The model under review builds one solid part; all positions refer to its coordinate system, in mm. A direction names the side the tool comes from. Coordinates: 2 decimals unless noted, no trailing zeros. Write each loop counter-clockwise with the first axis right and the second up, starting at its lowest first coordinate (ties: lowest second). Pieces come first, ordered by that corner, then holes. Notation, with made-up numbers: (26, 9) - (61, 9) arc R8 cw to (61, 20) - close; hole circle Ø2 at (51, -0.5). An arc over 180 degrees is marked (long way). Return JSON: item names as keys, results as strings. Group by question number.
(1) For pin 1 Ø3 at (x, y) = (108, -9.5) entering from +Z; pin 2 Ø9 at (y, z) = (0.5, -7) entering from +X; pin 3 Ø1 at (x, y) = (56.5, 34) entering from -Z; pin 4 Ø5 at (x, z) = (20, -49.5) entering from +Y, all flat-tipped, find the tip position at first contact; note any pin that passes through.
(2) We need section A-A on y = 0. Give the number of separate pieces and of enclosed holes in the cut face, then the cut area to 3 significant figures.
(3) To check wall thickness, follow L1, parallel to Z at x = 16.5, y = 0; L2, parallel to Y at x = 63.5, z = 4.5; L3, parallel to Z at x = 56, y = -7.5. State the ranges of each line that lie inside material, in increasing order. Write a range as from..to.
(4) Draft analysis for pull direction Y (two halves, no side actions). For faces 1 (the face through (15.653, 34.918, -3.952)), 2 (the face through (46.64, -49.76, -38.16)), 3 (the face through (0, -1, 1)), state which applies: released by +Y, released by -Y, zero draft, split by the parting line, or undercut.
(5) Tool access review of faces 4 (the face through (57.506, -56.413, -9.173)), 5 (the face through (171.45, 0, 0)): name each direction out of +Z, -Z, +X, -X, +Y, -Y from which nothing blocks a thin tool from reaching the whole face with its end or side.
(6) We need section B-B on x = 46.5. State the section outline as (y, z) points.
```python
from build123d import *

# Parameters (mm, degrees)
F0_R            = 73.025
F1_DEPTH        = 12.7
F2_R            = 62.70625
F3_DEPTH        = 69.85
F4_R            = 15.875
F5_DEPTH        = 25.4
F6_R            = 7
F7_DEPTH        = 63.5
F8_SIZE         = 1.016
F9_SIZE         = 1.524
F11_D           = 20.6375
F11_CBORE_D     = 30.1498
F11_CBORE_DEPTH = 50.8


# Not quite as in the source:
# - a length typed as a fraction of an inch, garbled in the dataset ("3 / 203.2 mm" for 3/8 in), is restored


with BuildPart() as f1:
    # F0 (on Right) → F1 (new body)
    with BuildSketch(Plane.YZ):
        Circle(F0_R)
    extrude(amount=F1_DEPTH)

    # F2 (on face) → F3 (join)
    with BuildSketch(Plane.YZ.offset(12.7)):
        Circle(F2_R)
    extrude(amount=F3_DEPTH)

    # F4 (on face) → F5 (join)
    with BuildSketch(Plane.YZ.offset(82.55)):
        Circle(F4_R)
    extrude(amount=F5_DEPTH)

    # F6 (on face) → F7 (join)
    with BuildSketch(Plane.YZ.offset(107.95)):
        Circle(F6_R)
    extrude(amount=F7_DEPTH)

    # F8
    f8_edges = [f1.edges().sort_by_distance(p)[0] for p in [
        (6.35, 73.025, 0),
        (0, -73.025, 0),
        (12.7, -73.025, 0),
        (82.55, -62.70625, 0),
        (107.95, -15.875, 0),
    ]]
    chamfer(f8_edges, length=F8_SIZE)

    # F9
    f9_edges = [f1.edges().sort_by_distance(p)[0] for p in [
        (171.45, -7, 0),
    ]]
    chamfer(f9_edges, length=F9_SIZE)

    # F11 (through all)
    with Locations(Plane.YZ.offset(82.55)):
        with Locations((0, 44.45), (44.45, 0), (0, -44.45), (-44.45, 0)):
            CounterBoreHole(F11_D / 2, F11_CBORE_D / 2, F11_CBORE_DEPTH)


solid = f1.part
```
Ans:
{
 "1": {"pin 1": "z = 13.44", "pin 2": "x = 171.45", "pin 3": "z = -53.01", "pin 4": "y = 41.51"},
 "2": {"separate pieces": "3", "enclosed holes": "0", "area": "7,930 mm²"},
 "3": {"L1": "-62.71..-54.77, -34.13..34.13, 54.77..62.71", "L2": "-62.54..-58.84, -30.06..30.06, 58.84..62.54", "L3": "-62.26..-57.53, -31.37..31.37, 57.53..62.26"},
 "4": {"face 1": "undercut", "face 2": "split by the parting line", "face 3": "zero draft"},
 "5": {"face 4": "+X", "face 5": "+Z, -Z, +X, +Y, -Y"},
 "6": {"outline": "circle Ø125.41 at (0, 0); hole circle Ø30.15 at (-44.45, 0); hole circle Ø30.15 at (0, -44.45); hole circle Ø30.15 at (0, 44.45); hole circle Ø30.15 at (44.45, 0)"}
}
